The drawing under review shows one solid part. Ordinate dimensions are in mm from its lowest x, y, z. Coordinates: 2 decimals unless noted, no trailing zeros. Order: outer loops, then holes, each group sorted by start corner. A loop starts at its lowest first (then second) coordinate and runs counter-clockwise, first axis right, second up. Notation, with made-up numbers: (1, 33) -> (13, 33) arc R13 ccw to (13, 56) -> close; hole circle Ø6 at (11, 87.25). An arc over 180 degrees is marked (long way). Write item = value, one per line.
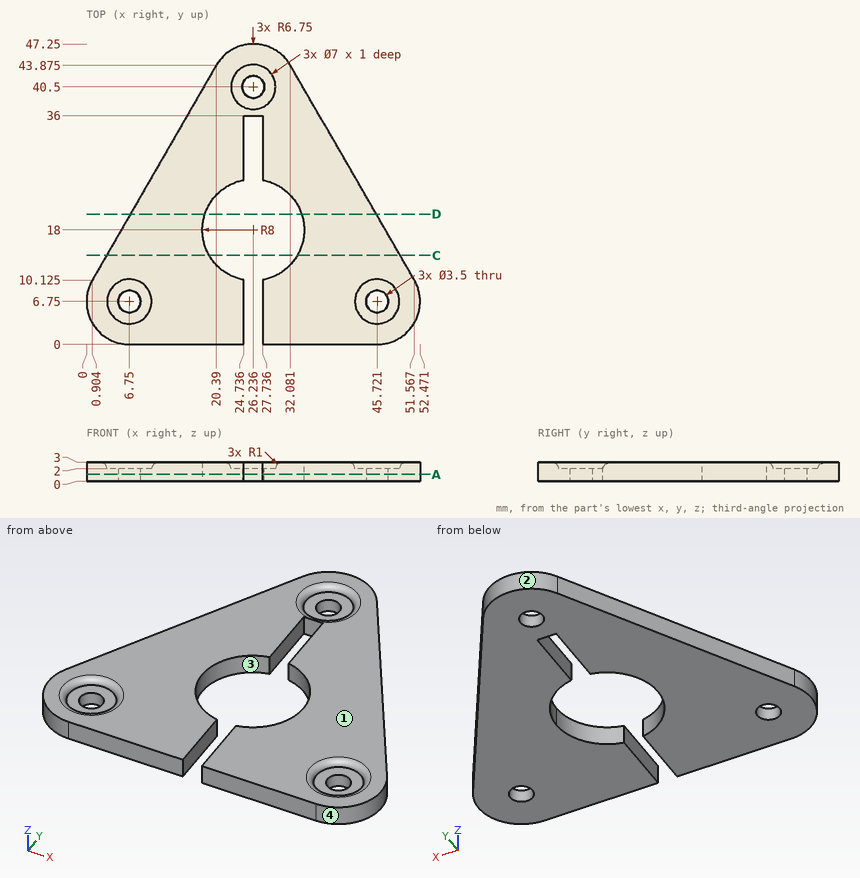
(1) Insertion check: pin 1 (0.9 mm diameter, centred on y = 32, z = 1.5, fed in from -X) (1 decimal); pin 2 (3.5 mm diameter, centred on x = 44, y = 5.5, fed in from +Z); pin 3 (1.5 mm diameter, centred on y = 3, z = 1, fed in from +X). Each pin has a flat end and moves straight along its axis. Give the tip position at first contact, or say it passes through.
Report:
pin_1 = 13.3
pin_2 = 2.78
pin_3 = 51.77
(2) We need section D-D (y = 20.5). Write out the cut boundary in (x, z) (1 decimal).
Report:
outline = (6.9, 0) -> (18.6, 0) -> (18.6, 3) -> (6.9, 3) -> close; (33.8, 0) -> (45.6, 0) -> (45.6, 3) -> (33.8, 3) -> close
(3) For L1, parallel to X at y = 6.75, z = 0.6 (1 decimal); L2, parallel to X at y = 8, z = 0.2 (1 decimal); L3, parallel to Y at x = 27.5, z = 2.1, list the stretches that pass through material, from the lowest coordinate up.
Report:
L1 = 0 to 5, 8.5 to 24.7, 27.7 to 44, 47.5 to 52.5
L2 = 0.1 to 5.5, 8 to 24.7, 27.7 to 44.5, 46.9 to 52.4
L3 = 36 to 37.23, 43.77 to 47.13
(4) We need section C-C (y = 14). Write out the cut boundary in (x, z).
Report:
outline = (3.14, 0) -> (19.31, 0) -> (19.31, 3) -> (3.14, 3) -> close; (33.16, 0) -> (49.33, 0) -> (49.33, 3) -> (33.16, 3) -> close
(5) We need section A-A (z = 1.1). Give the number of separate pieces and of enclosed holes in the cut face, and give its area (3 significant figures).
Report:
separate_pieces = 1
enclosed_holes = 3
area = 1,300 mm²
(6) The part is to be moulded in two halves that separate along X. For the marked faces 1, 2, 3 and 4, say which applies: released by +X, released by -X, zero draft, split by the parting line, or undercut.
Report:
face_1 = zero draft
face_2 = split by the parting line
face_3 = undercut
face_4 = released by +X
